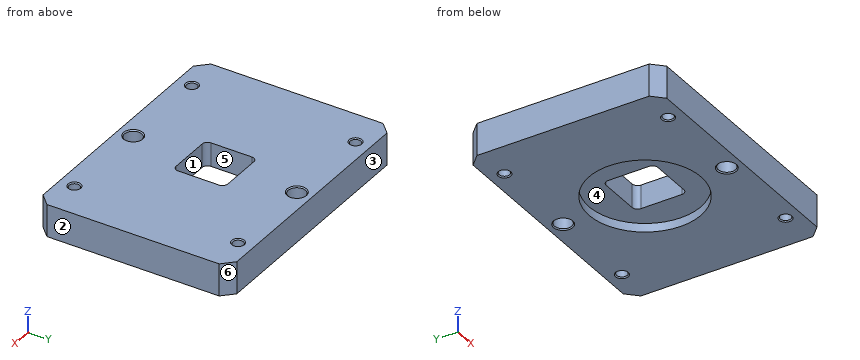
Solid Edge part; units mm, degrees
sketch "Sketch1" plane through (0, 0, 0) normal (0, 0, 1) x (1, 0, 0)
  line L0 (-60, -45) -> (60, -45)
  line L1 (60, -45) -> (60, 45)
  line L2 (60, 45) -> (-60, 45)
  line L3 (-60, 45) -> (-60, -45)
extrude "Protrusion1" add sketch "Sketch1" along normal blind 15
sketch "Sketch2" plane through (0, 0, 0) normal (0, 0, -1) x (1, 0, 0)
  circle A0 centre (0, 0) radius 26
extrude "VaciadoExtruido_1" cut sketch "Sketch2" against normal blind 4
sketch "Sketch3" plane through (0, 0, 4) normal (0, 0, -1) x (1, 0, 0)
  line L0 (-12, -12) -> (12, -12)
  line L1 (12, -12) -> (12, 12)
  line L2 (12, 12) -> (-12, 12)
  line L3 (-12, 12) -> (-12, -12)
  dimension "D1" = 12
  dimension "D2" = 12
extrude "Cutout1" cut sketch "Sketch3" against normal through all
fillet "Redondeo_1" radius 2.5 4 edges at (-12, 12, 9.5) (-12, -12, 9.5) (12, -12, 9.5) (12, 12, 9.5)
chamfer "Chaflán_1" distance 5 angle 45 4 edges at (-60, 45, 7.5) (-60, -45, 7.5) (60, -45, 7.5) (60, 45, 7.5)
hole "Agujero_1" at (0, 38, 15) direction (0, 0, -1) diameter 8 end up to next start chamfer 0.5 start chamfer angle 45 end chamfer 0.5 end chamfer angle 45
hole "Hole1" at (0, -38, 15) direction (0, 0, -1) diameter 8 end up to next start chamfer 0.5 start chamfer angle 45 end chamfer 0.5 end chamfer angle 45
hole "Hole2" at (43, -38, 15) direction (0, 0, -1) diameter 4.917 end through all start chamfer 0.5 start chamfer angle 45 end chamfer 0.5 end chamfer angle 45
hole "Hole3" at (-43, -38, 15) direction (0, 0, -1) diameter 4.917 end through all start chamfer 0.5 start chamfer angle 45 end chamfer 0.5 end chamfer angle 45
hole "Hole4" at (-43, 38, 15) direction (0, 0, -1) diameter 4.917 end through all start chamfer 0.5 start chamfer angle 45 end chamfer 0.5 end chamfer angle 45
hole "Hole5" at (43, 38, 15) direction (0, 0, -1) diameter 4.917 end through all start chamfer 0.5 start chamfer angle 45 end chamfer 0.5 end chamfer angle 45
properties part number "1976-1200-001" material "Aluminio, 7075-T6"
Verification items for the finished model (mm, model axes). Face numbers are marked on the shaded views. A direction names the side the tool comes from. Coordinates: 2 decimals unless noted, no trailing zeros. Write each loop counter-clockwise with the first axis right and the second up, starting at its lowest first coordinate (ties: lowest second). Pieces come first, ordered by that corner, then holes. Notation, with made-up numbers: M -4.75,60.5 L 25.25,60.5 A18 ccw 25.25,93.5 Z; hole C -1.5,-35.75 d9. An arc over 180 degrees is marked long. One line per question, with ' | ' between items.
1) Sectioned sample at B-B on y = -38. Record the cut outline in (x, z), then the cut area to 3 significant figures.
Solutions:
outline: M -60,0 L -45.96,0 L -45.46,0.5 L -45.46,14.5 L -45.96,15 L -60,15 Z; M -40.54,0.5 L -40.04,0 L -4.5,0 L -4,0.5 L -4,14.5 L -4.5,15 L -40.04,15 L -40.54,14.5 Z; M 4,0.5 L 4.5,0 L 40.04,0 L 40.54,0.5 L 40.54,14.5 L 40.04,15 L 4.5,15 L 4,14.5 Z; M 45.46,0.5 L 45.96,0 L 60,0 L 60,15 L 45.96,15 L 45.46,14.5 Z | area: 1,530 mm^2
2) Release check for a two-part mould opening along Y. For the marked faces 1, 2 and 3 record: +Y half, -Y half, draft (parallel to the pull), parting line (faces both ways), or undercut.
Solutions:
face 1: undercut | face 2: draft | face 3: +Y half
3) Depth check by flat-ended pin: pin 1 Ø7 at (x, y) = (0, -38) entering from -Z. Enter the tip coordinate at first touch or a pass-through.
Solutions:
pin 1: through
4) Sectioned sample at A-A on x = -43. Record the cut outline in (y, z), then the cut area to 3 significant figures.
Solutions:
outline: M -45,0 L -40.96,0 L -40.46,0.5 L -40.46,14.5 L -40.96,15 L -45,15 Z; M -35.54,0.5 L -35.04,0 L 35.04,0 L 35.54,0.5 L 35.54,14.5 L 35.04,15 L -35.04,15 L -35.54,14.5 Z; M 40.46,0.5 L 40.96,0 L 45,0 L 45,15 L 40.96,15 L 40.46,14.5 Z | area: 1,200 mm^2
5) Sectioned sample at C-C on x = 0. Record the cut outline in (y, z).
Solutions:
outline: M -45,0 L -42.5,0 L -42,0.5 L -42,14.5 L -42.5,15 L -45,15 Z; M -34,0.5 L -33.5,0 L -26,0 L -26,4 L -12,4 L -12,15 L -33.5,15 L -34,14.5 Z; M 12,4 L 26,4 L 26,0 L 33.5,0 L 34,0.5 L 34,14.5 L 33.5,15 L 12,15 Z; M 42,0.5 L 42.5,0 L 45,0 L 45,15 L 42.5,15 L 42,14.5 Z
6) Material ranges on L1, parallel to X at y = -38, z = 5.25; L2, parallel to Y at x = -43, z = 10.25; L3, parallel to X at y = 0, z = 1.3, recorded low to high.
Solutions:
L1: -60 to -45.46, -40.54 to -4, 4 to 40.54, 45.46 to 60 | L2: -45 to -40.46, -35.54 to 35.54, 40.46 to 45 | L3: -60 to -26, 26 to 60
7) Sectioned sample at D-D on y = 0. Record the cut outline in (x, z), then the cut area to 3 significant figures.
Solutions:
outline: M -60,0 L -26,0 L -26,4 L -12,4 L -12,15 L -60,15 Z; M 12,4 L 26,4 L 26,0 L 60,0 L 60,15 L 12,15 Z | area: 1,330 mm^2
8) Access from +Z, -Z, +X, -X, +Y, -Y to the whole of each face (thin tool, end or side, straight path). Record for the marked faces 4, 5 and 6.
Solutions:
face 4: -Z | face 5: +Z, -Z | face 6: +Z, -Z, +X, +Y
